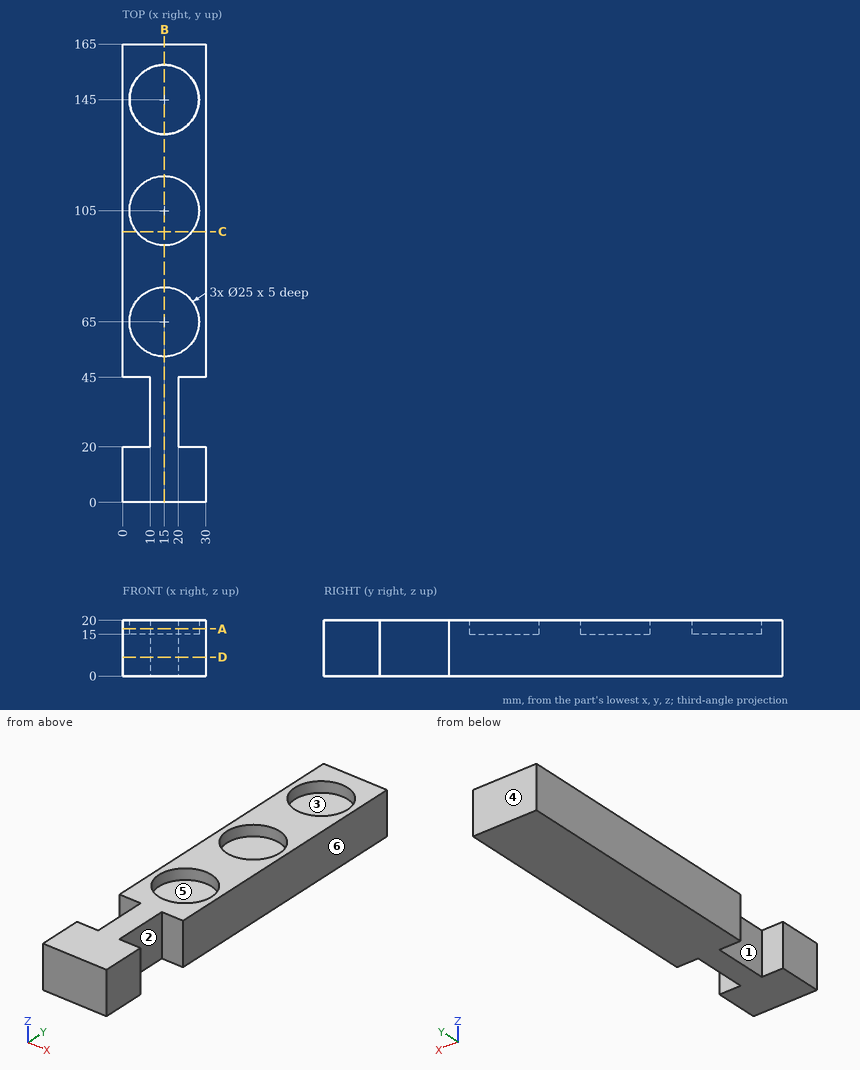
For this review, use the dimensioned drawing (mm, ordinates from the lowest corner) and the shaded views. A direction names the side the tool comes from. Coordinates: 2 decimals unless noted, no trailing zeros. Loops run counter-clockwise (first coordinate to the right, second up) from the corner with the lowest first, then second, coordinate; pieces in that order, holes last. Notation, with made-up numbers: (-5, -2) -> (54, -2) arc R35 cw to (54, 32) -> close; hole circle Ø10 at (-25.75, 39.5). An arc over 180 degrees is marked (long way). Use a Markdown table: item, result. Add a question column.
Item 1: We need section A-A, the plane z = 17. Write out the cut boundary in (x, y), and give its area (3 significant figures).
Item 2: We need section D-D, the plane z = 6.75. Write out the cut boundary in (x, y), and give its area (3 significant figures).
Item 3: Wall thickness on L1, parallel to Y at x = 15, z = 16.35; L2, parallel to Y at x = 7, z = 14.25; L3, parallel to X at y = 105, z = 16.3: over which ranges is each line inside the solid? List them lowest first. Write a range as from..to.
Item 4: Clearance check with flat-ended pins moving along their axes: P1, Ø10, axis at y = 32, z = 11.5, coming from the +X side; P2, Ø12.5, axis at x = 11, y = 66, coming from the +Z side; P3, Ø10, axis at y = 38, z = 7.5, coming from the -X side. State where each tip first meets the part, or that it passes through.
Item 5: We need section B-B, the plane x = 15. Write out the cut boundary in (y, z).
Item 6: We need section C-C, the plane y = 97.5. Write out the cut boundary in (x, z).
Item 7: The part is to be moulded in two halves that separate along Y. For the marked faces 4, 5 and 6, say which applies: +Y half, -Y half, draft (parallel to the pull), parting line (faces both ways), or undercut.
Item 8: Machinability: for the marked faces 1, 2 and 3, which of the approach directions +Z, -Z, +X, -X, +Y, -Y give a long, thin tool a straight path to every point of the face, cutting with its end or side? Answer none if there is none.
Numbers:
| question | item | result |
|---|---|---|
| 1 | outline | (0, 0) -> (30, 0) -> (30, 20) -> (20, 20) -> (20, 45) -> (30, 45) -> (30, 165) -> (0, 165) -> (0, 45) -> (10, 45) -> (10, 20) -> (0, 20) -> close; hole circle Ø25 at (15, 65); hole circle Ø25 at (15, 105); hole circle Ø25 at (15, 145) |
| 1 | area | 2,980 mm^2 |
| 2 | outline | (0, 0) -> (30, 0) -> (30, 20) -> (20, 20) -> (20, 45) -> (30, 45) -> (30, 165) -> (0, 165) -> (0, 45) -> (10, 45) -> (10, 20) -> (0, 20) -> close |
| 2 | area | 4,450 mm^2 |
| 3 | L1 | y = 0..52.5, 77.5..92.5, 117.5..132.5, 157.5..165 |
| 3 | L2 | y = 0..20, 45..165 |
| 3 | L3 | x = 0..2.5, 27.5..30 |
| 4 | P1 | stops at x = 20 |
| 4 | P2 | stops at z = 15 |
| 4 | P3 | stops at x = 10 |
| 5 | outline | (0, 0) -> (165, 0) -> (165, 20) -> (157.5, 20) -> (157.5, 15) -> (132.5, 15) -> (132.5, 20) -> (117.5, 20) -> (117.5, 15) -> (92.5, 15) -> (92.5, 20) -> (77.5, 20) -> (77.5, 15) -> (52.5, 15) -> (52.5, 20) -> (0, 20) -> close |
| 6 | outline | (0, 0) -> (30, 0) -> (30, 20) -> (25, 20) -> (25, 15) -> (5, 15) -> (5, 20) -> (0, 20) -> close |
| 7 | face 4 | +Y half |
| 7 | face 5 | undercut |
| 7 | face 6 | draft |
| 8 | face 1 | +Z, -Z, -X |
| 8 | face 2 | +Z, -Z, +X |
| 8 | face 3 | +Z |
